from build123d import *

# Parameters (mm, degrees)
BOSS_EXTRUDE1_DEPTH     = 1.5
CUT_EXTRUDE1_DEPTH      = 33.580828274
CUT_EXTRUDE1_DEPTH_BACK = 33.580828274
SKETCH2_R               = 1.75
CHAMFER2_SIZE           = 1
CHAMFER4_SIZE           = 1


with BuildPart() as part:
    # Sketch1 → Boss-Extrude1 (new body)
    with BuildSketch(Plane(origin=(0, 0, 0), x_dir=(1, 0, 0), z_dir=(0, 1, 0))):
        Polygon((21.25, 17.848471223), (-21.25, 17.848471223), (-21.25, 4.848471223), (-6.5, 4.848471223), (-6.5, -24.651528777), (6.5, -24.651528777), (6.5, 4.848471223), (21.25, 4.848471223), align=None)
    extrude(amount=BOSS_EXTRUDE1_DEPTH)

    # Sketch2 → Cut-Extrude1 (cut, two sides: drawn at the far end of the back side and taken through both)
    with BuildSketch(Plane(origin=(0, 1.5, 0), x_dir=(1, 0, 0), z_dir=(0, 1, 0)).offset(-CUT_EXTRUDE1_DEPTH_BACK)):
        with Locations(Location((-13.756799801, 11.348471223, 0), (0, 0, 270))):
            Circle(SKETCH2_R)
        with Locations(Location((13.756799801, 11.348471223, 0), (0, 0, 90))):
            Circle(SKETCH2_R)
        with Locations(Location((0, -2.526528777, 0), (0, 0, 270))):
            Circle(SKETCH2_R)
        with Locations(Location((0, -17.276528777, 0), (0, 0, 90))):
            Circle(SKETCH2_R)
    extrude(amount=CUT_EXTRUDE1_DEPTH + CUT_EXTRUDE1_DEPTH_BACK, mode=Mode.SUBTRACT)

    # Chamfer2
    chamfer2_edges = [part.edges().sort_by_distance(p)[0] for p in [
        (-13.756799801, 1.5, -13.098471223),
    ]]
    chamfer(chamfer2_edges, length=CHAMFER2_SIZE)

    # Chamfer4
    chamfer4_edges = [part.edges().sort_by_distance(p)[0] for p in [
        (13.756799801, 1.5, -9.598471223),
        (0, 1.5, 19.026528777),
        (0, 1.5, 0.776528777),
    ]]
    chamfer(chamfer4_edges, length=CHAMFER4_SIZE)


solid = part.part
Verification items for the finished model (mm, model axes). A direction names the side the tool comes from. Coordinates: 2 decimals unless noted, no trailing zeros. Loops run counter-clockwise (first coordinate to the right, second up) from the corner with the lowest first, then second, coordinate; pieces in that order, holes last. Notation, with made-up numbers: (63.5, 10) -> (68.5, 10) arc R10 ccw to (68.5, 18) -> close; hole circle Ø8 at (-39.5, -40). An arc over 180 degrees is marked (long way). Answer as a JSON object with one key per item and string values. Group by question number.
Item 1: Sectioned sample at B-B on y = 1.1. Record the boundary of the cut face in (x, z), plus the area to 3 significant figures.
Item 2: Sectioned sample at A-A on x = 0. Record the boundary of the cut face in (y, z), plus the area to 4 significant figures.
Item 3: Mould release check, pull along Z, two halves, no side actions. Record for faces 4 (the flat face through (-6.5, 1, 10)), 5 (the flat face through (0, 1, 24.652)), 6 (the cylindrical face through (14.82, 0.25, -9.96)): +Z half, -Z half, draft (parallel to the pull), parting line (faces both ways), or undercut.
Item 4: Sectioned sample at D-D on z = 13.5. Record the boundary of the cut face in (x, y).
Item 5: Sectioned sample at C-C on x = -8. Record the boundary of the cut face in (y, z).
Item 6: Tool access check on faces 1 (the flat face through (14, 1, -4.848)), 2 (the cylindrical face through (0.08, 0.25, 0.78)), 3 (the flat face through (-14, 1, -4.848)). Record the directions out of +Z, -Z, +X, -X, +Y, -Y that give a thin tool (end or side, any length) a straight path to the whole face; none if there is none.
Item 7: Scan lines: probe 1 along X at (y, z) = (0.65, -13); probe 2 along X at (y, z) = (1.1, -4.5); probe 3 along X at (y, z) = (0.2, 2.5). Record each from-to range of solid material in increasing order.
Item 8: Depth check by flat-ended pin: pin 1 (4.5 mm diameter, centred on x = -13.76, z = -11.35, fed in from -Y). Enter the tip coordinate at first touch or a pass-through.
Evaluation:
{
 "1": {"outline": "(-21.25, -17.85) -> (21.25, -17.85) -> (21.25, -4.85) -> (6.5, -4.85) -> (6.5, 24.65) -> (-6.5, 24.65) -> (-6.5, -4.85) -> (-21.25, -4.85) -> close; hole circle Ø4.7 at (-13.76, -11.35); hole circle Ø4.7 at (0, 2.53); hole circle Ø4.7 at (0, 17.28); hole circle Ø4.7 at (13.76, -11.35)", "area": "867 mm²"},
 "2": {"outline": "(0, -17.85) -> (1.5, -17.85) -> (1.5, -0.22) -> (0.5, 0.78) -> (0, 0.78) -> close; (0, 4.28) -> (0.5, 4.28) -> (1.5, 5.28) -> (1.5, 14.53) -> (0.5, 15.53) -> (0, 15.53) -> close; (0, 19.03) -> (0.5, 19.03) -> (1.5, 20.03) -> (1.5, 24.65) -> (0, 24.65) -> close", "area": "51.25 mm²"},
 "3": {"face 4": "draft", "face 5": "+Z half", "face 6": "undercut"},
 "4": {"outline": "(-6.5, 0) -> (6.5, 0) -> (6.5, 1.5) -> (-6.5, 1.5) -> close"},
 "5": {"outline": "(0, -17.85) -> (1.5, -17.85) -> (1.5, -4.85) -> (0, -4.85) -> close"},
 "6": {"face 1": "+Z, +X, +Y, -Y", "face 2": "+Y, -Y", "face 3": "+Z, -X, +Y, -Y"},
 "7": {"probe 1": "x = -21.25 to -14.7, -12.82 to 12.82, 14.7 to 21.25", "probe 2": "x = -6.5 to 6.5", "probe 3": "x = -6.5 to -1.75, 1.75 to 6.5"},
 "8": {"pin 1": "stops at y = 0"}
}
